```python
from build123d import *

# Parameters (mm, degrees)
CHANFREIN1_SIZE              = 1
TROU_TARAUD_M81_REACH        = 76.682
TROU_TARAUD_M81_BORE_R       = 3.4
ENL_V_MAT_EXTRU_1_DEPTH      = 66.543878463
ENL_V_MAT_EXTRU_1_DEPTH_BACK = 66.543878463
ESQUISSE4_W                  = 8
ESQUISSE4_H                  = 2.832418839


with BuildPart() as part:
    # Esquisse1 → Révolution1 (revolve)
    with BuildSketch(Plane.XY, mode=Mode.PRIVATE) as r_volution1_sk:
        Polygon((-14.5, 4), (-14.5, 10), (0, 10), (0, 7.5), (64, 7.5), (64, 0), (6.165063509, 0), (4, 3.75), (2, 3.75), (2, 4), align=None)
    revolve(r_volution1_sk.sketch.rotate(Axis((-22.202680924, 0, 0), (1, 0, 0)), 90), axis=Axis((-22.202680924, 0, 0), (1, 0, 0)))

    # Chanfrein1
    chanfrein1_edges = [part.edges().sort_by_distance(p)[0] for p in [
        (64, 0, -7.5),
        (-14.5, 0, -10),
    ]]
    chamfer(chanfrein1_edges, length=CHANFREIN1_SIZE)

    # Trou taraudé M81 bore (on position points) → Trou taraudé M81 (cut, up to next)
    with BuildSketch(Plane(origin=(-7.255410761, 0, 10), x_dir=(1, 0, 0), z_dir=(0, 0, 1)), mode=Mode.PRIVATE) as trou_taraud_m81_sk1:
        Circle(TROU_TARAUD_M81_BORE_R)
    trou_taraud_m81_tool1 = extrude(trou_taraud_m81_sk1.sketch, amount=-TROU_TARAUD_M81_REACH, mode=Mode.PRIVATE) & part.part
    add(trou_taraud_m81_tool1.solids().sort_by_distance((-7.255411, 0, 10))[0], mode=Mode.SUBTRACT)

    # Esquisse4 → Enlèv. mat.-Extru.1 (cut, two sides: drawn at the far end of the back side and taken through both)
    with BuildSketch(Plane(origin=(0, 0, 0), x_dir=(1, 0, 0), z_dir=(0, 1, 0)).offset(-ENL_V_MAT_EXTRU_1_DEPTH_BACK)):
        with Locations((48, -7.91620942)):
            Rectangle(ESQUISSE4_W, ESQUISSE4_H)
    extrude(amount=ENL_V_MAT_EXTRU_1_DEPTH + ENL_V_MAT_EXTRU_1_DEPTH_BACK, mode=Mode.SUBTRACT)


solid = part.part
```
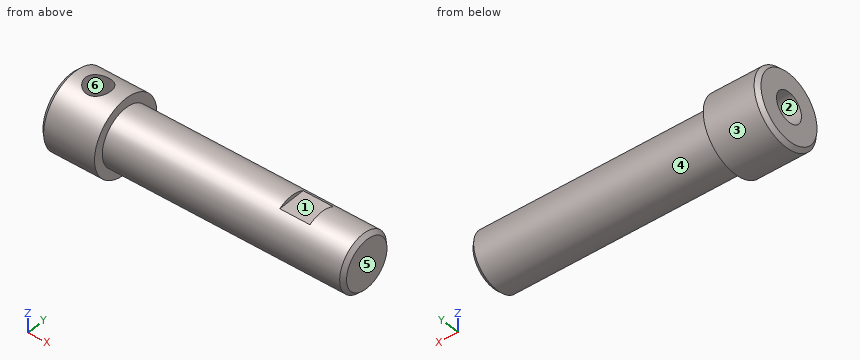
Verification items for the finished model (mm, model axes). Face numbers are marked on the shaded views. A direction names the side the tool comes from. Coordinates: 2 decimals unless noted, no trailing zeros. Loops run counter-clockwise (first coordinate to the right, second up) from the corner with the lowest first, then second, coordinate; pieces in that order, holes last. Notation, with made-up numbers: (13.5, 16) -> (18.5, 16) arc R20 ccw to (18.5, 31) -> close; hole circle Ø2 at (-26.75, 49.25). An arc over 180 degrees is marked (long way). Answer in a Markdown table with one row per item. Add a question column.
1. Section check B-B, the plane x = 40.5. Enter the section's corners in (y, z).
2. Section check A-A, the plane x = 3. Enter the section's corners in (y, z).
3. Access from +Z, -Z, +X, -X, +Y, -Y to the whole of each face (thin tool, end or side, straight path). Record for the marked faces 4, 5 and 6.
4. Depth check by flat-ended pin: P1, Ø8, axis at y = -0.5, z = 1.5, coming from the -X side; P2, Ø8, axis at x = 10, z = -4, coming from the -Y side; P3, Ø8, axis at x = 16, y = 6.5, coming from the -Z side; P4, Ø2, axis at x = 45.5, z = 2.5, coming from the -Y side. Enter the tip coordinate at first touch or a pass-through.
5. Draft check along Y on the marked faces 1, 2 and 3. Enter one of: +Y half, -Y half, draft (parallel to the pull), parting line (faces both ways), or undercut.
6. Material ranges on probe 1 along Y at (x, z) = (3.15, 0); probe 2 along X at (y, z) = (-0.5, 4); probe 3 along Z at (x, y) = (-5.5, 3.25), recorded low to high. Write a range as [from, to].
Derived:
| question | item | result |
|---|---|---|
| 1 | outline | circle Ø15 at (0, 0) |
| 2 | outline | circle Ø15 at (0, 0); hole circle Ø7.5 at (0, 0) |
| 3 | face 4 | +X |
| 3 | face 5 | +Z, -Z, +X, +Y, -Y |
| 3 | face 6 | +Z |
| 4 | P1 | stops at x = -14.5 |
| 4 | P2 | stops at y = -7.5 |
| 4 | P3 | stops at z = -7.07 |
| 4 | P4 | stops at y = -7.35 |
| 5 | face 1 | draft |
| 5 | face 2 | undercut |
| 5 | face 3 | parting line |
| 6 | probe 1 | y = [-7.5, -3.75], [3.75, 7.5] |
| 6 | probe 2 | x = [-14.5, -10.62], [-3.89, 64] |
| 6 | probe 3 | z = [-9.46, -2.33], [2.33, 9.46] |
